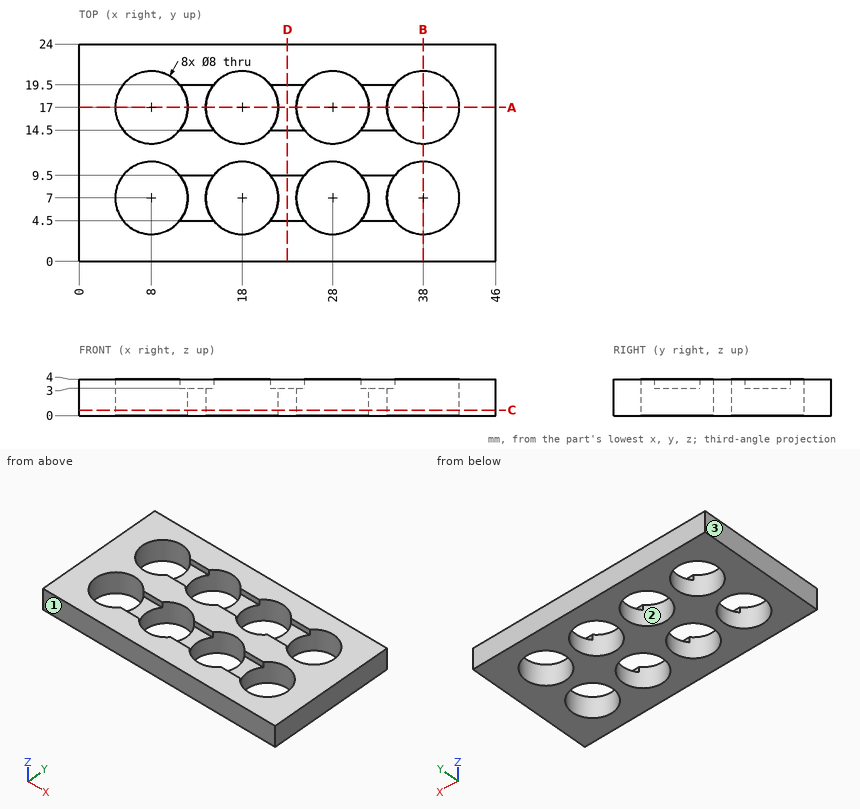
Job drawing, mm, ordinate dimensions from the low corner. One solid piece. Coordinates: 2 decimals unless noted, no trailing zeros. Write each loop counter-clockwise with the first axis right and the second up, starting at its lowest first coordinate (ties: lowest second). Pieces come first, ordered by that corner, then holes.
Item 1: Slice it at C-C (z = 0.6). Count the separate pieces of the cut face and the enclosed holes in it, and give its area (3 significant figures).
Item 2: Slice it at B-B (x = 38). Write the cut outline in (y, z), and give its area (3 significant figures).
Item 3: Probe line 1 (Y direction, x = 38, z = 1.9); line 2 (X direction, y = 7, z = 1.35); line 3 (X direction, y = 6, z = 1.9). List the from-to ranges inside material, lowest first.
Item 4: Mould opens along Y. For the marked faces 1, 2 and 3 say: released by +Y, released by -Y, zero draft, split by the parting line, or undercut.
Item 5: Slice it at D-D (x = 23). Write the cut outline in (y, z).
Item 6: Slice it at A-A (y = 17). Write the cut outline in (x, z), and give its area (3 significant figures).
Item 7: Pin check, flat tips, straight feed: pin 1 (1.9 mm diameter, centred on x = 13.5, y = 8, fed in from +Z); pin 2 (6.5 mm diameter, centred on x = 18, y = 7, fed in from +Z). Stop position of each tip, or through.
Results found:
1. separate pieces: 1
1. enclosed holes: 8
1. area: 702 mm2
2. outline: (0, 0) - (3, 0) - (3, 4) - (0, 4) - close; (11, 0) - (13, 0) - (13, 4) - (11, 4) - close; (21, 0) - (24, 0) - (24, 4) - (21, 4) - close
2. area: 32.0 mm2
3. line 1: y = 0 to 3, 11 to 13, 21 to 24
3. line 2: x = 0 to 4, 12 to 14, 22 to 24, 32 to 34, 42 to 46
3. line 3: x = 0 to 4.13, 11.87 to 14.13, 21.87 to 24.13, 31.87 to 34.13, 41.87 to 46
4. face 1: released by -Y
4. face 2: undercut
4. face 3: zero draft
5. outline: (0, 0) - (24, 0) - (24, 4) - (19.5, 4) - (19.5, 3) - (14.5, 3) - (14.5, 4) - (9.5, 4) - (9.5, 3) - (4.5, 3) - (4.5, 4) - (0, 4) - close
6. outline: (0, 0) - (4, 0) - (4, 4) - (0, 4) - close; (12, 0) - (14, 0) - (14, 3) - (12, 3) - close; (22, 0) - (24, 0) - (24, 3) - (22, 3) - close; (32, 0) - (34, 0) - (34, 3) - (32, 3) - close; (42, 0) - (46, 0) - (46, 4) - (42, 4) - close
6. area: 50.0 mm2
7. pin 1: stops at z = 3
7. pin 2: passes through
